Autodesk Inventor part; units mm, degrees
ref_plane "YZ Plane" through (0, 0, 0) normal (1, 0, 0) x (0, 1, 0)
ref_plane "XZ Plane" through (0, 0, 0) normal (0, 1, 0) x (-1, 0, 0)
ref_plane "XY Plane" through (0, 0, 0) normal (0, 0, 1) x (1, 0, 0)
sketch "Sketch1" plane through (0, 0, 0) normal (0, 0, 1) x (1, 0, 0)
  line L0 (21, -21) -> (-21, -21)
  line L1 (-21, -21) -> (-21, 21)
  line L2 (-21, 21) -> (21, 21)
  line L3 (21, 21) -> (21, -21)
  line L4 (21, -21) -> (-21, 21) construction
  line L5 (-21, -21) -> (21, 21) construction
  point P0 (0, 0)
  dimension "d0" = 42
extrude "Extrusion1" add sketch "Sketch1" along normal blind 34
chamfer "Chamfer1" distance 3.5 angle 45 4 edges at (-21, 21, 17) (21, 21, 17) (21, -21, 17) (-21, -21, 17)
sketch "Sketch2" plane through (0, 0, 34) normal (0, 0, 1) x (1, 0, 0)
  circle A0 centre (0, 0) radius 11
  dimension "d6" = 22
extrude "Extrusion2" add sketch "Sketch2" along normal blind 2
sketch "Sketch3" plane through (0, 0, 36) normal (0, 0, 1) x (1, 0, 0)
  circle A0 centre (0, 0) radius 4
  dimension "d9" = 8
extrude "Extrusion3" add sketch "Sketch3" along normal blind 363
thread "Thread1"
chamfer "Chamfer2" distance 1 angle 45 1 edges at (-4, 0, 399)
sketch "Sketch4" plane through (0, 0, 34) normal (0, 0, 1) x (1, 0, 0)
  line L0 (-17.5, -21) -> (17.5, -21)
  line L1 (17.5, 21) -> (-17.5, 21)
  line L2 (-21, 17.5) -> (-21, -17.5)
  point P0 (0, 0)
  point P1 (-15.5, 15.5)
  point P2 (-15.5, -15.5)
  point P3 (15.5, -15.5)
  point P4 (15.5, 15.5)
  dimension "d17" = 31
  dimension "d18" = 31
  dimension "d19" = 42
  dimension "d21" = 5.5
  dimension "d22" = 5.5
hole "Hole1" at (-15.5, 15.5, 34) at (-15.5, -15.5, 34) at (15.5, -15.5, 34) at (15.5, 15.5, 34) direction (0, 0, -1) diameter 2.459 depth 8.8 tip angle 118
properties part number "Motor_Z" material "Steel, Alloy"
Check sheet for the modelled part. Datum: model origin and axes. Units: mm. A direction names the side the tool comes from. Round coordinates to 2 decimals unless told otherwise and drop trailing zeros. Loops run counter-clockwise (first coordinate to the right, second up) from the corner with the lowest first, then second, coordinate; pieces in that order, holes last. Notation, with made-up numbers: M -20,-19 L 32,-19 A13 ccw 32,6 Z; hole C -7,5.25 d5. An arc over 180 degrees is marked long. One line per question, with ' | ' between items. Start each with the question number.
Item 1: Section check A-A (z = 251). Record the boundary of the cut face in (x, y).
Item 2: Scan lines: probe 1 along Y at (x, z) = (15.5, 30.5); probe 2 along Y at (x, z) = (-15, 29). Record each from-to range of solid material in increasing order.
Item 3: Gauge pin test, flat ends, axial feed: pin 1 Ø10 at (y, z) = (-13, 256) entering from -X; pin 2 Ø10 at (y, z) = (-7.5, 339.5) entering from +X; pin 3 Ø4 at (x, y) = (15.5, 15.5) entering from +Z; pin 4 Ø3 at (x, z) = (4, 192.5) entering from -Y. Record the tip position at first contact, or that the pin passes through.
Item 4: Set-up check for faces 1 (the face through (0, 0, 0)), 2 (the face through (-0.867, 3.905, 214.466)): record each of +Z, -Z, +X, -X, +Y, -Y from which the full face is reachable in a straight line by a thin tool's end or side.
Worked out:
1) outline: C 0,0 d8
2) probe 1: -21 to -16.73, -14.27 to 14.27, 16.73 to 21 | probe 2: -21 to -16.62, -14.38 to 14.38, 16.62 to 21
3) pin 1: through | pin 2: x = 3.12 | pin 3: z = 34 | pin 4: y = -3.12
4) face 1: -Z, +X, -X, +Y, -Y | face 2: +Z
